Autodesk Inventor part; units mm, degrees
ref_plane "YZ Plane" through (0, 0, 0) normal (1, 0, 0) x (0, 1, 0)
ref_plane "XZ Plane" through (0, 0, 0) normal (0, 1, 0) x (-1, 0, 0)
ref_plane "XY Plane" through (0, 0, 0) normal (0, 0, 1) x (1, 0, 0)
sketch "Sketch3" plane through (0, 0, 0) normal (0, 0, 1) x (1, 0, 0)
  line L0 (13.0384, -3.5) -> (21.0384, -3.5)
  line L1 (-13.0384, 3.5) -> (-21.0384, 3.5)
  line L2 (0, 13.5) -> (28, 13.5)
  line L3 (0, -13.5) -> (-28, -13.5)
  arc A0 (-21.0384, 3.5) -> (-28, -13.5) centre (11.5082, -19.7534) ccw
  arc A1 (21.0384, -3.5) -> (28, 13.5) centre (-11.5082, 19.7534) ccw
  arc A2 (0, 13.5) -> (-13.0384, 3.5) centre (0, 0) ccw
  arc A3 (0, -13.5) -> (13.0384, -3.5) centre (0, 0) ccw
  circle A4 centre (0, 0) radius 2.5
  dimension "d29" = 8
  dimension "d30" = 8
  dimension "d33" = 28
  dimension "d34" = 28
  dimension "d35" = 40
  dimension "d36" = 40
  dimension "d37" = 5
extrude "Extrusion2" add sketch "Sketch3" along normal blind 3
properties part number "ArmaPrime"
Check sheet for the modelled part. Datum: model origin and axes. Units: mm. Coordinates: 2 decimals unless noted, no trailing zeros. Order: outer loops, then holes, each group sorted by start corner. A loop starts at its lowest first (then second) coordinate and runs counter-clockwise, first axis right, second up. Notation, with made-up numbers: (65, 8) -> (87, 8) arc R24 cw to (87, 43) -> close; hole circle Ø2 at (63, 23). An arc over 180 degrees is marked (long way). Write item = value, one per line. Start each with the question number.
1) Cross-section at B-B (y = 0). Enter the section's corners in (x, z), then the cut area to 3 significant figures.
2) Go/stop test with flat-tipped pins: P1, Ø5, axis at x = 20.5, y = -6.5, coming from the -Z side; P2, Ø1, axis at y = -5, z = 2, coming from the +X side. Record where each tip stops, or that it passes through.
3) Cross-section at C-C (y = 7.75). Enter the section's corners in (x, z).
4) Mould release check, pull along Y, two halves, no side actions. Record for faces 1 (the flat face through (17, -3.5, 1)), 2 (the flat face through (-17, 3.5, 1)), 3 (the cylindrical face through (-0.54, 2.44, 1.48)): +Y half, -Y half, draft (parallel to the pull), parting line (faces both ways), or undercut.
5) Cross-section at A-A (z = 0.45). Enter the section's corners in (x, y), then the cut area to 3 significant figures.
6) Material ranges on L1, parallel to Y at x = 0, z = 1.8; L2, parallel to Y at x = -15.5, z = 2.4; L3, parallel to Y at x = 19, z = 1.35, recorded low to high.
7) Cross-section at D-D (y = -7.25). Enter the section's corners in (x, z).
Ans:
q1.outline = (-23.27, 0) -> (-2.5, 0) -> (-2.5, 3) -> (-23.27, 3) -> close; (2.5, 0) -> (23.27, 0) -> (23.27, 3) -> (2.5, 3) -> close
q1.area = 125 mm²
q2.P1 = through
q2.P2 = 12.73
q3.outline = (-11.05, 0) -> (26.65, 0) -> (26.65, 3) -> (-11.05, 3) -> close
q4.face_1 = -Y half
q4.face_2 = +Y half
q4.face_3 = undercut
q5.outline = (-28, -13.5) -> (0, -13.5) arc R13.5 ccw to (13.04, -3.5) -> (21.04, -3.5) arc R40 ccw to (28, 13.5) -> (0, 13.5) arc R13.5 ccw to (-13.04, 3.5) -> (-21.04, 3.5) arc R40 ccw to start; hole circle Ø5 at (0, 0)
q5.area = 1,030 mm²
q6.L1 = -13.5 to -2.5, 2.5 to 13.5
q6.L2 = -13.5 to 3.5
q6.L3 = -3.5 to 13.5
q7.outline = (-26.49, 0) -> (11.39, 0) -> (11.39, 3) -> (-26.49, 3) -> close
